Build history of the part. All positions in model axes, mm. Face numbers are marked on the shaded views. Give positions to 0.01 mm unless a question says otherwise; leave off trailing zeros. Loops run counter-clockwise (first coordinate to the right, second up) from the corner with the lowest first, then second, coordinate; pieces in that order, holes last. Notation, with made-up numbers: M 68,-15.5 L 102,-15.5 A20 ccw 102,16.5 Z; hole C 28,-30 d4. An arc over 180 degrees is marked long. Answer in a Markdown table with one row per item. Add a question column.
```python
from build123d import *

# Parameters (mm, degrees)
SKETCH1_R           = 2.2
BOSS_EXTRUDE1_DEPTH = 4
SKETCH2_W           = 5
SKETCH2_H           = 5
BOSS_EXTRUDE2_DEPTH = 8
FILLET1_R           = 8


with BuildPart() as part:
    # Sketch1 → Boss-Extrude1 (new body)
    with BuildSketch(Plane.XY):
        with BuildLine():
            Line((-30, 0), (30, 0))
            Line((30, 0), (30, 5))
            ThreePointArc((30, 5), (13.861944355, 10.296039854), (4, 24.124522477))
            Line((4, 24.124522477), (4, 96))
            ThreePointArc((4, 96), (0, 100), (-4, 96))
            Line((-4, 96), (-4, 24.124522477))
            ThreePointArc((-4, 24.124522477), (-13.861944355, 10.296039854), (-30, 5))
            Line((-30, 5), (-30, 0))
        make_face()
        with Locations((0, 96)):
            Circle(SKETCH1_R, mode=Mode.SUBTRACT)
        with BuildLine():
            Line((-14.576406349, 4.5), (14.576406349, 4.5))
            ThreePointArc((14.576406349, 4.5), (5.681813978, 11.844889874), (0, 21.883723005))
            ThreePointArc((0, 21.883723005), (-5.681813978, 11.844889874), (-14.576406349, 4.5))
        make_face(mode=Mode.SUBTRACT)
    extrude(amount=BOSS_EXTRUDE1_DEPTH)

    # Sketch2 → Boss-Extrude2 (add)
    with BuildSketch(Plane.XY.offset(4)):
        with Locations((27.5, 2.5)):
            Rectangle(SKETCH2_W, SKETCH2_H)
        with Locations((-27.5, 2.5)):
            Rectangle(SKETCH2_W, SKETCH2_H)
    extrude(amount=BOSS_EXTRUDE2_DEPTH)

    # Fillet1
    # the kernel refuses this fillet: 8 mm, written as the material it takes off along each edge
    with BuildSketch(Plane(origin=(6.459503782, 5, 12), x_dir=(0, -1, 0), z_dir=(1, 0, 0))) as fillet1_piece_1:
        with BuildLine():
            CenterArc((8, 7.416198487), FILLET1_R, 180, 67.975687163)
            Line((0, 7.416198487), (-0.16, 7.416198487))
            Line((-0.16, 7.416198487), (-0.16, 0))
            Line((-0.16, 0), (0, -0.16))
            ThreePointArc((0, -0.16), (2.5, -0.16), (4.94, -0.14832397))
            Line((4.94, -0.14832397), (5, 0))
        make_face()
    extrude(amount=42.080992435, mode=Mode.SUBTRACT)
    with BuildSketch(Plane(origin=(-6.459503782, 5, 12), x_dir=(0, 0, -1), z_dir=(-1, 0, 0))) as fillet1_piece_2:
        with BuildLine():
            CenterArc((7.416198487, 8), FILLET1_R, 202.024312837, 67.975687163)
            Line((0, 5), (-0.14832397, 4.94))
            ThreePointArc((-0.14832397, 4.94), (-0.16, 2.5), (-0.16, 0))
            Line((-0.16, 0), (0, -0.16))
            Line((0, -0.16), (7.416198487, -0.16))
            Line((7.416198487, -0.16), (7.416198487, 0))
        make_face()
    extrude(amount=42.080992435, mode=Mode.SUBTRACT)


solid = part.part
```
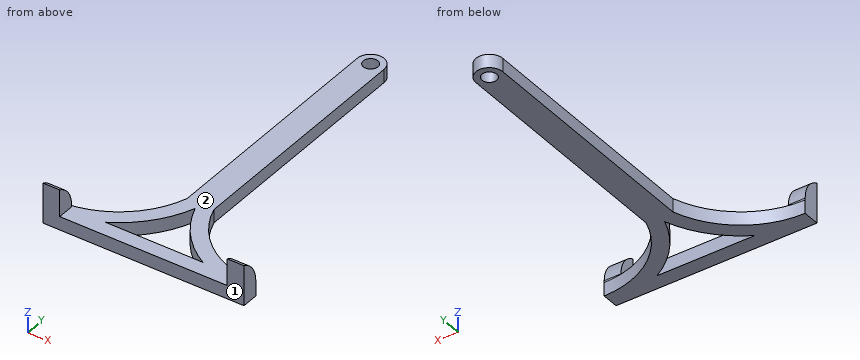
(1) Wall check: line 1 (X direction, y = 86, z = 3.75); line 2 (Y direction, x = -8.5, z = 0.75); line 3 (Z direction, x = 8, y = 11). Give the ranges that are in metal, low to high.
(2) Pin check, flat tips, straight feed: pin 1 (3 mm diameter, centred on y = 52.5, z = 2.5, fed in from -X); pin 2 (3.5 mm diameter, centred on x = 0, y = 96, fed in from +Z); pin 3 (6 mm diameter, centred on x = -3.5, y = 84.5, fed in from +Z); pin 4 (1.2 mm diameter, centred on y = 70.5, z = 1, fed in from +X). Stop position of each tip, or through.
(3) Slice it at D-D, the plane x = -22. Give the cut face in (y, z), then the cut area to 3 significant figures.
(4) Slice it at B-B, the plane x = 12.5. Give the cut face in (y, z).
(5) Pull direction X, two halves, no side cores. Call the marked faces 1 and 2: +X half, -X half, draft (parallel to the pull), parting line (faces both ways), or undercut.
(6) Slice it at A-A, the plane z = 10.75. Give the cut face in (x, y).
(7) Slice it at C-C, the plane y = 63. Give the cut face in (x, z).
Solution:
| question | item | result |
|---|---|---|
| 1 | line 1 | -4 to 4 |
| 1 | line 2 | 0 to 4.5, 8.89 to 15.52 |
| 1 | line 3 | 0 to 4 |
| 2 | pin 1 | x = -4 |
| 2 | pin 2 | through |
| 2 | pin 3 | z = 4 |
| 2 | pin 4 | x = 4 |
| 3 | outline | M 0,0 L 6.2,0 L 6.2,4 L 0,4 Z |
| 3 | area | 24.8 mm^2 |
| 4 | outline | M 0,0 L 4.5,0 L 4.5,4 L 0,4 Z; M 5.76,0 L 11.37,0 L 11.37,4 L 5.76,4 Z |
| 5 | face 1 | draft |
| 5 | face 2 | undercut |
| 6 | outline | M -30,0 L -25,0 L -25,2.1 L -30,2.1 Z; M 25,0 L 30,0 L 30,2.1 L 25,2.1 Z |
| 7 | outline | M -4,0 L 4,0 L 4,4 L -4,4 Z |
